```python
from build123d import *

# Parameters (mm, degrees)
F0_W     = 80
F0_H     = 45
F1_DEPTH = 1.5
F2_W     = 76.4
F2_H     = 41.4
F2_W_2   = 73.4
F2_H_2   = 38.4
F3_DEPTH = 1.5
F5_DEPTH = 76.4
F6_DEPTH = 76.4


with BuildPart() as f1:
    # F0 (on Top) → F1 (new body)
    with BuildSketch(Plane.XY):
        with Locations((0.812615, 2.5)):
            Rectangle(F0_W, F0_H)
        with BuildLine():
            ThreePointArc((-8.437385, 0), (-9.321268, 0.366117), (-9.687385, 1.25))
            Line((-9.687385, 1.25), (-9.687385, 3.75))
            ThreePointArc((-9.687385, 3.75), (-9.321268, 4.633883), (-8.437385, 5))
            ThreePointArc((-8.437385, 5), (-7.553501, 4.633883), (-7.187385, 3.75))
            Line((-7.187385, 3.75), (-7.187385, 1.25))
            ThreePointArc((-7.187385, 1.25), (-7.553501, 0.366117), (-8.437385, 0))
        make_face(mode=Mode.SUBTRACT)
        with BuildLine():
            ThreePointArc((-3.437385, -1.5), (-4.321268, -1.133883), (-4.687385, -0.25))
            Line((-4.687385, -0.25), (-4.687385, 5.25))
            ThreePointArc((-4.687385, 5.25), (-4.321268, 6.133883), (-3.437385, 6.5))
            ThreePointArc((-3.437385, 6.5), (-2.553501, 6.133883), (-2.187385, 5.25))
            Line((-2.187385, 5.25), (-2.187385, -0.25))
            ThreePointArc((-2.187385, -0.25), (-2.553501, -1.133883), (-3.437385, -1.5))
        make_face(mode=Mode.SUBTRACT)
        with BuildLine():
            ThreePointArc((1.562615, -3.5), (0.678732, -3.133883), (0.312615, -2.25))
            Line((0.312615, -2.25), (0.312615, 7.25))
            ThreePointArc((0.312615, 7.25), (0.678732, 8.133883), (1.562615, 8.5))
            ThreePointArc((1.562615, 8.5), (2.446499, 8.133883), (2.812615, 7.25))
            Line((2.812615, 7.25), (2.812615, -2.25))
            ThreePointArc((2.812615, -2.25), (2.446499, -3.133883), (1.562615, -3.5))
        make_face(mode=Mode.SUBTRACT)
        with BuildLine():
            ThreePointArc((6.562615, -5), (5.678732, -4.633883), (5.312615, -3.75))
            Line((5.312615, -3.75), (5.312615, 8.75))
            ThreePointArc((5.312615, 8.75), (5.678732, 9.633883), (6.562615, 10))
            ThreePointArc((6.562615, 10), (7.446499, 9.633883), (7.812615, 8.75))
            Line((7.812615, 8.75), (7.812615, -3.75))
            ThreePointArc((7.812615, -3.75), (7.446499, -4.633883), (6.562615, -5))
        make_face(mode=Mode.SUBTRACT)
        with BuildLine():
            Line((10.312615, -6.25), (10.312615, 11.25))
            ThreePointArc((10.312615, 11.25), (10.678732, 12.133883), (11.562615, 12.5))
            ThreePointArc((11.562615, 12.5), (12.446499, 12.133883), (12.812615, 11.25))
            Line((12.812615, 11.25), (12.812615, -6.25))
            ThreePointArc((12.812615, -6.25), (12.446499, -7.133883), (11.562615, -7.5))
            ThreePointArc((11.562615, -7.5), (10.678732, -7.133883), (10.312615, -6.25))
        make_face(mode=Mode.SUBTRACT)
        with BuildLine():
            Line((14.812615, -8.75), (14.812615, 13.75))
            ThreePointArc((14.812615, 13.75), (15.178732, 14.633883), (16.062615, 15))
            ThreePointArc((16.062615, 15), (16.946499, 14.633883), (17.312615, 13.75))
            Line((17.312615, 13.75), (17.312615, -8.75))
            ThreePointArc((17.312615, -8.75), (16.946499, -9.633883), (16.062615, -10))
            ThreePointArc((16.062615, -10), (15.178732, -9.633883), (14.812615, -8.75))
        make_face(mode=Mode.SUBTRACT)
        with BuildLine():
            Line((19.312615, -11.25), (19.312615, 16.25))
            ThreePointArc((19.312615, 16.25), (19.678732, 17.133883), (20.562615, 17.5))
            ThreePointArc((20.562615, 17.5), (21.446499, 17.133883), (21.812615, 16.25))
            Line((21.812615, 16.25), (21.812615, -11.25))
            ThreePointArc((21.812615, -11.25), (21.446499, -12.133883), (20.562615, -12.5))
            ThreePointArc((20.562615, -12.5), (19.678732, -12.133883), (19.312615, -11.25))
        make_face(mode=Mode.SUBTRACT)
        with BuildLine():
            Line((23.812615, -11.25), (23.812615, 16.25))
            ThreePointArc((23.812615, 16.25), (24.178732, 17.133883), (25.062615, 17.5))
            ThreePointArc((25.062615, 17.5), (25.946499, 17.133883), (26.312615, 16.25))
            Line((26.312615, 16.25), (26.312615, -11.25))
            ThreePointArc((26.312615, -11.25), (25.946499, -12.133883), (25.062615, -12.5))
            ThreePointArc((25.062615, -12.5), (24.178732, -12.133883), (23.812615, -11.25))
        make_face(mode=Mode.SUBTRACT)
        with BuildLine():
            Line((28.312615, -8.75), (28.312615, 13.75))
            ThreePointArc((28.312615, 13.75), (28.678732, 14.633883), (29.562615, 15))
            ThreePointArc((29.562615, 15), (30.446499, 14.633883), (30.812615, 13.75))
            Line((30.812615, 13.75), (30.812615, -8.75))
            ThreePointArc((30.812615, -8.75), (30.446499, -9.633883), (29.562615, -10))
            ThreePointArc((29.562615, -10), (28.678732, -9.633883), (28.312615, -8.75))
        make_face(mode=Mode.SUBTRACT)
        with BuildLine():
            Line((32.812615, -6.25), (32.812615, 11.25))
            ThreePointArc((32.812615, 11.25), (33.178732, 12.133883), (34.062615, 12.5))
            ThreePointArc((34.062615, 12.5), (34.946499, 12.133883), (35.312615, 11.25))
            Line((35.312615, 11.25), (35.312615, -6.25))
            ThreePointArc((35.312615, -6.25), (34.946499, -7.133883), (34.062615, -7.5))
            ThreePointArc((34.062615, -7.5), (33.178732, -7.133883), (32.812615, -6.25))
        make_face(mode=Mode.SUBTRACT)
    extrude(amount=F1_DEPTH)

    # F2 (on face) → F3 (join)
    with BuildSketch(Plane(origin=(0, 0, 0), x_dir=(1, 0, 0), z_dir=(0, 0, -1))):
        with Locations((0.812615, -2.5)):
            Rectangle(F2_W, F2_H)
        with Locations((0.812615, -2.5)):
            Rectangle(F2_W_2, F2_H_2, mode=Mode.SUBTRACT)
    extrude(amount=F3_DEPTH)

    # F4 (on face) → F5 (join)
    with BuildSketch(Plane.YZ.offset(39.012615)):
        Polygon((23.7, -3.847339), (23.2, -1.5), (22.2, -1.5), (22.7, -3.847339), align=None)
    extrude(amount=-F5_DEPTH)

    # F4 (on face) → F6 (join)
    with BuildSketch(Plane.YZ.offset(39.012615)):
        Polygon((23.7, -3.847339), (23.2, -1.5), (22.2, -1.5), (22.7, -3.847339), align=None)
        Polygon((-18.7, -3.847339), (-17.7, -3.847339), (-17.2, -1.5), (-18.2, -1.5), align=None)
    extrude(amount=-F6_DEPTH)


solid = f1.part
```
Geometry check sheet. Reference: the model listing, model coordinates, mm. A direction names the side the tool comes from. Coordinates: 2 decimals unless noted, no trailing zeros. Loops run counter-clockwise (first coordinate to the right, second up) from the corner with the lowest first, then second, coordinate; pieces in that order, holes last.
Item 1: Sectioned sample at B-B, the plane x = -15.5. Record the boundary of the cut face in (y, z).
Item 2: Sectioned sample at A-A, the plane z = -2.8. Record the boundary of the cut face in (x, y), then the cut area to 3 significant figures.
Item 3: Release check for a two-part mould opening along X. For faces 1 (the face through (35.313, 3, 1)), 2 (the face through (-2, -19, 0)), 3 (the face through (-37.387, 2, -1)) record: released by +X, released by -X, zero draft, split by the parting line, or undercut.
Item 4: Thickness scan on line 1 (X direction, y = -1.5, z = -1); line 2 (Y direction, x = -30.5, z = -0.5); line 3 (Y direction, x = 34, z = 0.5). Record the ranges inside material, lowest first.
Item 5: Access from +Z, -Z, +X, -X, +Y, -Y to the whole of each face (thin tool, end or side, straight path). Record for faces 4 (the face through (-8, 7, 0)), 5 (the face through (10.313, 2, 1)), 6 (the face through (39.013, 2, -1)).
Item 6: Go/stop test with flat-tipped pins: pin 1 Ø1.2 at (x, z) = (-9.5, -1) entering from +Y; pin 2 Ø1 at (y, z) = (17.5, -3) entering from -X; pin 3 Ø8 at (x, y) = (-3.5, 3.5) entering from -Z; pin 4 Ø1.5 at (x, z) = (12.5, -3) entering from +Y. Record where each tip stops, or that it passes through.
Check result:
1. outline: (-20, 0) - (-18.2, 0) - (-18.2, -1.5) - (-18.7, -3.85) - (-17.7, -3.85) - (-17.2, -1.5) - (-16.7, -1.5) - (-16.7, 0) - (21.7, 0) - (21.7, -1.5) - (22.2, -1.5) - (22.7, -3.85) - (23.7, -3.85) - (23.2, -1.5) - (23.2, 0) - (25, 0) - (25, 1.5) - (-20, 1.5) - close
2. outline: (-37.39, -18.48) - (39.01, -18.48) - (39.01, -17.48) - (-37.39, -17.48) - close; (-37.39, 22.48) - (39.01, 22.48) - (39.01, 23.48) - (-37.39, 23.48) - close
2. area: 153 mm2
3. face 1: undercut
3. face 2: zero draft
3. face 3: released by -X
4. line 1: x = -37.39 to -35.89, 37.51 to 39.01
4. line 2: y = -18.2 to -16.7, 21.7 to 23.2
4. line 3: y = -20 to -7.5, 12.5 to 25
5. face 4: -Z
5. face 5: +Z, -Z
5. face 6: -Z, +X, +Y, -Y
6. pin 1: stops at y = 23.22
6. pin 2: passes through
6. pin 3: stops at z = 0
6. pin 4: stops at y = 23.68
